Could you check a few things on this model? Use its own coordinates, in mm. Face numbers are marked on the shaded views. A direction names the side the tool comes from. Round coordinates to 2 decimals unless told otherwise and drop trailing zeros. Loops run counter-clockwise (first coordinate to the right, second up) from the corner with the lowest first, then second, coordinate; pieces in that order, holes last. Notation, with made-up numbers: (-34.5, 58) -> (-7.5, 58) arc R13 cw to (-7.5, 77) -> close; hole circle Ø7 at (66.5, -22). An arc over 180 degrees is marked (long way). Put each result on its own line as item: value. Start each with the question number.
1. If we mould it in two halves opening along Y, with no side actions, what happens to the marked faces 3, 4 and 5? For each: pulls with the +Y half, pulls with the -Y half, needs draft (parallel to the pull), parting line crosses it, or undercut.
2. Imagine slicing it at B-B, the plane y = 0. Please give me the cut outline in (x, z), and give its area (3 significant figures).
3. Imagine slicing it at D-D, the plane x = -12. Please give me the cut outline in (y, z).
4. I'm going to push flat-ended pins straight in: P1, Ø3, axis at x = 0, y = 6.5, coming from the -Z side; P2, Ø5, axis at x = 9, z = 3, coming from the +Y side; P3, Ø2, axis at y = -5.5, z = 8, coming from the -X side; P4, Ø5, axis at x = 10.5, z = -1.5, coming from the -Y side. Where does each tip first touch, or does it pass through?
5. Imagine slicing it at A-A, the plane x = 0. Please give me the cut outline in (y, z), and give its area (3 significant figures).
6. Imagine slicing it at C-C, the plane y = 6.5. Please give me the cut outline in (x, z), and give its area (3 significant figures).
7. I need wall thicknesses on line 1 (Y direction, x = 0, z = 7.8); line 2 (Z direction, x = -13, y = -14.5); line 3 (X direction, y = 18.5, z = 1). Which ranges of each line are inside material? Lowest first, please. Write a range as [from, to].
8. Which directions (+Z, -Z, +X, -X, +Y, -Y) give clear straight access to the entire face, cutting with the end or side of a thin tool? Please do the marked faces 1 and 2.
```python
from build123d import *

# Parameters (mm, degrees)
SKETCH1_R           = 30
BOSS_EXTRUDE1_DEPTH = 10.5
SKETCH2_R           = 1.55
SKETCH2_R_2         = 4
CUT_EXTRUDE1_DEPTH  = 10
SKETCH3_R           = 21
CUT_EXTRUDE2_DEPTH  = 17


with BuildPart() as part:
    # Sketch1 → Boss-Extrude1 (new, symmetric)
    with BuildSketch(Plane.XY):
        with Locations(Location((0, 0, 0), (0, 0, 180))):
            Circle(SKETCH1_R)
    extrude(amount=BOSS_EXTRUDE1_DEPTH, both=True)

    # Sketch2 → Cut-Extrude1 (cut)
    with BuildSketch(Plane.XY.offset(10.5)):
        with Locations((-6, 0)):
            Circle(SKETCH2_R)
        with Locations((0, 6.5)):
            Circle(SKETCH2_R)
        with Locations((6, 0)):
            Circle(SKETCH2_R)
        with Locations((0, -6.5)):
            Circle(SKETCH2_R)
        Circle(SKETCH2_R_2)
    extrude(amount=-CUT_EXTRUDE1_DEPTH, mode=Mode.SUBTRACT)

    # Sketch3 → Cut-Extrude2 (cut)
    with BuildSketch(Plane(origin=(0, 0, -10.5), x_dir=(-1, 0, 0), z_dir=(0, 0, -1))):
        Circle(SKETCH3_R)
    extrude(amount=-CUT_EXTRUDE2_DEPTH, mode=Mode.SUBTRACT)


solid = part.part
```
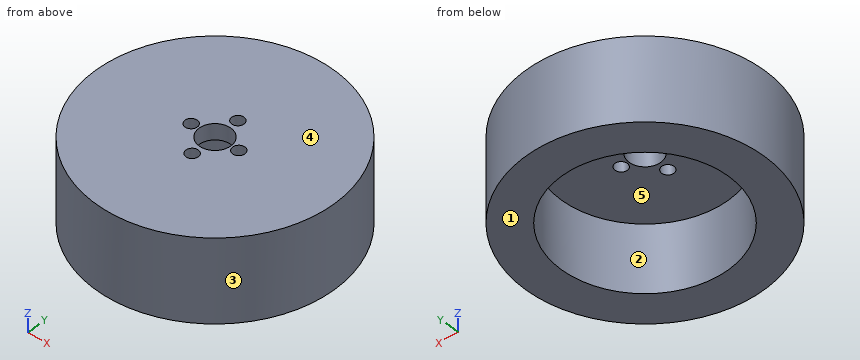
Entries:
1. face 3: parting line crosses it
1. face 4: needs draft
1. face 5: undercut
2. outline: (-30, -10.5) -> (-21, -10.5) -> (-21, 6.5) -> (-7.55, 6.5) -> (-7.55, 10.5) -> (-30, 10.5) -> close; (-4.45, 6.5) -> (-4, 6.5) -> (-4, 10.5) -> (-4.45, 10.5) -> close; (4, 6.5) -> (4.45, 6.5) -> (4.45, 10.5) -> (4, 10.5) -> close; (7.55, 6.5) -> (21, 6.5) -> (21, -10.5) -> (30, -10.5) -> (30, 10.5) -> (7.55, 10.5) -> close
2. area: 489 mm^2
3. outline: (-27.5, -10.5) -> (-17.23, -10.5) -> (-17.23, 6.5) -> (17.23, 6.5) -> (17.23, -10.5) -> (27.5, -10.5) -> (27.5, 10.5) -> (-27.5, 10.5) -> close
4. P1: through
4. P2: y = 29.29
4. P3: x = -29.66
4. P4: y = -28.91
5. outline: (-30, -10.5) -> (-21, -10.5) -> (-21, 6.5) -> (-8.05, 6.5) -> (-8.05, 10.5) -> (-30, 10.5) -> close; (-4.95, 6.5) -> (-4, 6.5) -> (-4, 10.5) -> (-4.95, 10.5) -> close; (4, 6.5) -> (4.95, 6.5) -> (4.95, 10.5) -> (4, 10.5) -> close; (8.05, 6.5) -> (21, 6.5) -> (21, -10.5) -> (30, -10.5) -> (30, 10.5) -> (8.05, 10.5) -> close
5. area: 489 mm^2
6. outline: (-29.29, -10.5) -> (-19.97, -10.5) -> (-19.97, 6.5) -> (-1.55, 6.5) -> (-1.55, 10.5) -> (-29.29, 10.5) -> close; (1.55, 6.5) -> (19.97, 6.5) -> (19.97, -10.5) -> (29.29, -10.5) -> (29.29, 10.5) -> (1.55, 10.5) -> close
6. area: 539 mm^2
7. line 1: [-30, -8.05], [-4.95, -4], [4, 4.95], [8.05, 30]
7. line 2: [6.5, 10.5]
7. line 3: [-23.62, -9.94], [9.94, 23.62]
8. face 1: -Z, +X, -X, +Y, -Y
8. face 2: -Z
